from build123d import *

# Parameters (mm, degrees)
SKETCH1_W           = 220
SKETCH1_H           = 120
SKETCH1_R           = 1.5
BOSS_EXTRUDE1_DEPTH = 5
SKETCH2_R           = 3.25
CUT_EXTRUDE1_DEPTH  = 5
SKETCH3_W           = 10
SKETCH3_H           = 10
CUT_EXTRUDE2_DEPTH  = 82.783407155
SKETCH4_W           = 10
SKETCH4_H           = 10
CUT_EXTRUDE3_DEPTH  = 5
FILLET1_R           = 2
SKETCH5_R           = 2
CUT_EXTRUDE4_DEPTH  = 5


with BuildPart() as part:
    # Sketch1 → Boss-Extrude1 (new body)
    with BuildSketch(Plane(origin=(0, 0, 0), x_dir=(1, 0, 0), z_dir=(0, 1, 0))):
        Rectangle(SKETCH1_W, SKETCH1_H)
        with Locations(Location((-22, 25, 0), (0, 0, 270))):
            Circle(SKETCH1_R, mode=Mode.SUBTRACT)
        with Locations(Location((-80, 25, 0), (0, 0, 90))):
            Circle(SKETCH1_R, mode=Mode.SUBTRACT)
        with Locations(Location((-22, -25, 0), (0, 0, 90))):
            Circle(SKETCH1_R, mode=Mode.SUBTRACT)
        with Locations(Location((-80, -25, 0), (0, 0, 270))):
            Circle(SKETCH1_R, mode=Mode.SUBTRACT)
        with Locations(Location((-2, 18.5, 0), (0, 0, 270))):
            Circle(SKETCH1_R, mode=Mode.SUBTRACT)
        with Locations(Location((35, 18.5, 0), (0, 0, 90))):
            Circle(SKETCH1_R, mode=Mode.SUBTRACT)
        with Locations(Location((35, -18.5, 0), (0, 0, 270))):
            Circle(SKETCH1_R, mode=Mode.SUBTRACT)
        with Locations(Location((-2, -18.5, 0), (0, 0, 90))):
            Circle(SKETCH1_R, mode=Mode.SUBTRACT)
        with Locations(Location((55, -18.5, 0), (0, 0, 90))):
            Circle(SKETCH1_R, mode=Mode.SUBTRACT)
        with Locations(Location((92, -18.5, 0), (0, 0, 270))):
            Circle(SKETCH1_R, mode=Mode.SUBTRACT)
        with Locations(Location((55, 18.5, 0), (0, 0, 270))):
            Circle(SKETCH1_R, mode=Mode.SUBTRACT)
        with Locations(Location((92, 18.5, 0), (0, 0, 90))):
            Circle(SKETCH1_R, mode=Mode.SUBTRACT)
    extrude(amount=BOSS_EXTRUDE1_DEPTH)

    # Sketch2 → Cut-Extrude1 (cut)
    with BuildSketch(Plane.XZ):
        with Locations(Location((56.593545043, -52.5, 0), (0, 0, 270))):
            Circle(SKETCH2_R)
        with Locations(Location((-86.593545043, -52.5, 0), (0, 0, 270))):
            Circle(SKETCH2_R)
        with Locations(Location((-86.593545043, 52.5, 0), (0, 0, 270))):
            Circle(SKETCH2_R)
        with Locations(Location((56.593545043, 52.5, 0), (0, 0, 270))):
            Circle(SKETCH2_R)
    extrude(amount=-CUT_EXTRUDE1_DEPTH, mode=Mode.SUBTRACT)

    # Sketch3 → Cut-Extrude2 (cut)
    with BuildSketch(Plane(origin=(0, 5, 0), x_dir=(1, 0, 0), z_dir=(0, 1, 0))):
        with Locations((5, -45)):
            Rectangle(SKETCH3_W, SKETCH3_H)
        with Locations((25, -45)):
            Rectangle(SKETCH3_W, SKETCH3_H)
        with Locations((25, 45)):
            Rectangle(SKETCH3_W, SKETCH3_H)
        with Locations((5, 45)):
            Rectangle(SKETCH3_W, SKETCH3_H)
    extrude(amount=-CUT_EXTRUDE2_DEPTH, mode=Mode.SUBTRACT)

    # Sketch4 → Cut-Extrude3 (cut)
    with BuildSketch(Plane(origin=(0, 5, 0), x_dir=(1, 0, 0), z_dir=(0, 1, 0))):
        with Locations((-34.127158997, -45)):
            Rectangle(SKETCH4_W, SKETCH4_H)
        with Locations((-34.127158997, 45)):
            Rectangle(SKETCH4_W, SKETCH4_H)
    extrude(amount=-CUT_EXTRUDE3_DEPTH, mode=Mode.SUBTRACT)

    # Fillet1
    fillet1_edges = [part.edges().sort_by_distance(p)[0] for p in [
        (0, 2.5, -50),
        (10, 2.5, -50),
        (10, 2.5, -40),
        (0, 2.5, -40),
        (30, 2.5, -50),
        (30, 2.5, -40),
        (30, 2.5, 40),
        (30, 2.5, 50),
        (20, 2.5, 50),
        (20, 2.5, 40),
        (0, 2.5, 50),
        (0, 2.5, 40),
        (10, 2.5, 40),
        (10, 2.5, 50),
        (-29.127158997, 2.5, 40),
        (-29.127158997, 2.5, 50),
        (-39.127158997, 2.5, 50),
        (-39.127158997, 2.5, 40),
        (-39.127158997, 2.5, -50),
        (-29.127158997, 2.5, -50),
        (-29.127158997, 2.5, -40),
        (-39.127158997, 2.5, -40),
        (-110, 2.5, -60),
        (110, 2.5, -60),
        (110, 2.5, 60),
        (-110, 2.5, 60),
    ]]
    fillet(fillet1_edges, radius=FILLET1_R)

    # Sketch5 → Cut-Extrude4 (cut)
    with BuildSketch(Plane(origin=(0, 5, 0), x_dir=(1, 0, 0), z_dir=(0, 1, 0))):
        with Locations(Location((88.15035354, -52.5, 0), (0, 0, 270))):
            Circle(SKETCH5_R)
        with Locations(Location((88.15035354, 52.5, 0), (0, 0, 270))):
            Circle(SKETCH5_R)
    extrude(amount=-CUT_EXTRUDE4_DEPTH, mode=Mode.SUBTRACT)


solid = part.part
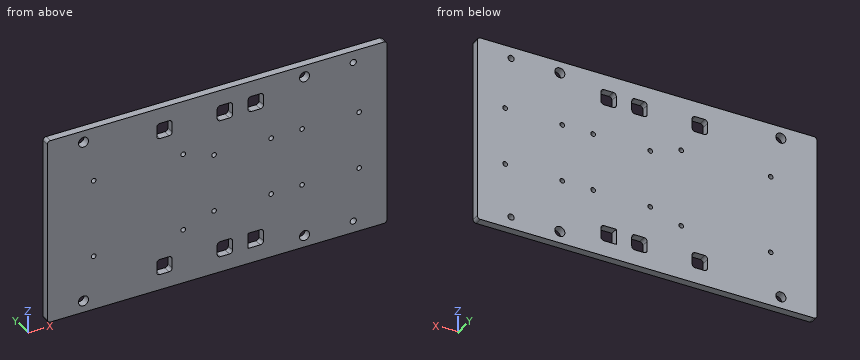
CAD build for the part. Positions are in the model's coordinates, mm. Coordinates: 2 decimals unless noted, no trailing zeros. Use a Markdown table: item, result. Add a question column.
Item 1: Band-saw the part on A-A, the plane y = 3.45. Give the number of separate pieces and of enclosed holes in the cut face, and give its area (3 significant figures).
Item 2: Flat gauge pin, fed straight in: pin 1 (2.5 mm diameter, centred on x = -22, z = 25, fed in from -Y). Where does the tip first touch, or does it go through?
Item 3: Drill centre lines: L1, parallel to X at y = 2.5, z = -25; L2, parallel to X at y = 1.5, z = 52.5; L3, parallel to X at y = 3.85, z = 41.5. Where is each one in solid material? Low to high. Write a range as from..to.
Numbers:
| question | item | result |
|---|---|---|
| 1 | separate pieces | 1 |
| 1 | enclosed holes | 24 |
| 1 | area | 25,600 mm2 |
| 2 | pin 1 | through |
| 3 | L1 | -110..-81.5, -78.5..-23.5, -20.5..110 |
| 3 | L2 | -110..-89.84, -83.34..53.34, 59.84..86.15, 90.15..110 |
| 3 | L3 | -110..-39.06, -29.19..0.06, 9.94..20.06, 29.94..110 |
